For this review, take the finished solid that the model builds, in its own axes (mm). Give positions to 0.01 mm unless a question says otherwise; leave off trailing zeros. Order: outer loops, then holes, each group sorted by start corner. A loop starts at its lowest first (then second) coordinate and runs counter-clockwise, first axis right, second up.
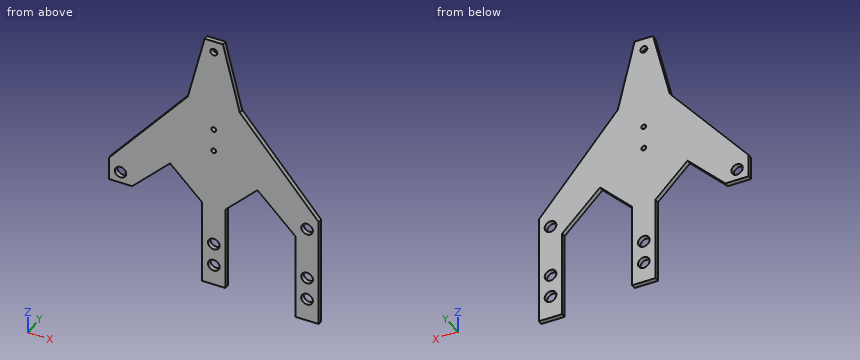
from build123d import *

# Parameters (mm, degrees)
SKETCH1_R           = 2.452812329
SKETCH1_R_2         = 2.5
SKETCH1_R_3         = 1.05
SKETCH1_R_4         = 1.5
BOSS_EXTRUDE1_DEPTH = 2


with BuildPart() as part:
    # Sketch1 → Boss-Extrude1 (new body)
    with BuildSketch(Plane(origin=(0, 0, 0), x_dir=(1, 0, 0), z_dir=(0, 1, 0))):
        Polygon((45, 45), (45, 35), (11.149880928, -5.279298766), (3.930911566, -35), (-3.930911566, -35), (-11.149880928, -5.279298766), (-45, 35), (-45, 45), (-35, 45), (-18.75, 28.75), (-5.004014664, 42.5), (-5.004014664, 79.531475099), (5, 79.531475099), (5, 42.5), (18.75, 28.75), (35, 45), (35, 83), (45, 83), align=None)
        with Locations(Location((-39.999958798, 40.081193315, 0), (0, 0, 270))):
            Circle(SKETCH1_R, mode=Mode.SUBTRACT)
        with Locations(Location((40, 40, 0), (0, 0, 270))):
            Circle(SKETCH1_R_2, mode=Mode.SUBTRACT)
        with Locations(Location((40, 63, 0), (0, 0, 270))):
            Circle(SKETCH1_R_2, mode=Mode.SUBTRACT)
        with Locations(Location((40, 73, 0), (0, 0, 270))):
            Circle(SKETCH1_R_2, mode=Mode.SUBTRACT)
        with Locations(Location((-0.004014664, 60.5, 0), (0, 0, 270))):
            Circle(SKETCH1_R_2, mode=Mode.SUBTRACT)
        with Locations(Location((0, 70.499999194, 0), (0, 0, 270))):
            Circle(SKETCH1_R_2, mode=Mode.SUBTRACT)
        with Locations(Location((0, 6.5, 0), (0, 0, 270))):
            Circle(SKETCH1_R_3, mode=Mode.SUBTRACT)
        with Locations(Location((0, 16.5, 0), (0, 0, 270))):
            Circle(SKETCH1_R_3, mode=Mode.SUBTRACT)
        with Locations(Location((0, -30, 0), (0, 0, 270))):
            Circle(SKETCH1_R_4, mode=Mode.SUBTRACT)
    extrude(amount=BOSS_EXTRUDE1_DEPTH)


solid = part.part
1) To check wall thickness, follow line 1 (X direction, y = 1, z = -76.5); line 2 (X direction, y = 1.4, z = -60); line 3 (X direction, y = 1, z = -16.5). State the ranges of each line that lie inside material, in increasing order.
Answer sheet:
line 1: x = -5 to 5, 35 to 45
line 2: x = -5 to -2.45, 2.45 to 5, 35 to 45
line 3: x = -29.45 to -1.05, 1.05 to 29.45
2) We need section C-C on y = 1.65. Count the separate pieces of the cut face and the enclosed holes in it, then the cut area to 3 significant figures.
Answer sheet:
separate pieces: 1
enclosed holes: 9
area: 3,680 mm2
3) We need section D-D on z = -39. Give the boundary of the cut face in (x, y), then the cut area to 3 significant figures.
Answer sheet:
outline: (-45, 0) - (-42.2, 0) - (-42.2, 2) - (-45, 2) - close; (-37.8, 0) - (-29, 0) - (-29, 2) - (-37.8, 2) - close; (-8.5, 0) - (8.5, 0) - (8.5, 2) - (-8.5, 2) - close; (29, 0) - (37.71, 0) - (37.71, 2) - (29, 2) - close; (42.29, 0) - (45, 0) - (45, 2) - (42.29, 2) - close
area: 80.0 mm2
4) Clearance check with flat-ended pins moving along their axes: pin 1 (4 mm diameter, centred on x = -40, z = -40.08, fed in from +Y); pin 2 (1.5 mm diameter, centred on x = 3, z = -11, fed in from -Y); pin 3 (1 mm diameter, centred on y = 1, z = -52.5, fed in from -X); pin 4 (1 mm diameter, centred on y = 1, z = 22, fed in from -X). State where each tip first meets the part, or that it passes through.
Answer sheet:
pin 1: passes through
pin 2: stops at y = 0
pin 3: stops at x = -5
pin 4: stops at x = -7.21
5) We need section A-A on z = 30. Give the boundary of the cut face in (x, y), then the cut area to 3 significant figures.
Answer sheet:
outline: (-5.15, 0) - (-1.5, 0) - (-1.5, 2) - (-5.15, 2) - close; (1.5, 0) - (5.15, 0) - (5.15, 2) - (1.5, 2) - close
area: 14.6 mm2
6) We need section B-B on x = 40. Give the boundary of the cut face in (y, z).
Answer sheet:
outline: (0, -83) - (2, -83) - (2, -75.5) - (0, -75.5) - close; (0, -70.5) - (2, -70.5) - (2, -65.5) - (0, -65.5) - close; (0, -60.5) - (2, -60.5) - (2, -42.5) - (0, -42.5) - close; (0, -37.5) - (2, -37.5) - (2, -29.05) - (0, -29.05) - close
